```python
from build123d import *

# Parameters (mm, degrees)
SKETCH1_W           = 123.84
SKETCH1_H           = 33
BOSS_EXTRUDE1_DEPTH = 10
SKETCH2_W           = 12
SKETCH2_H           = 57
BOSS_EXTRUDE2_DEPTH = 70
SKETCH3_R           = 23.5
CUT_EXTRUDE1_DEPTH  = 124.84
SKETCH10_R          = 45
BOSS_EXTRUDE5_DEPTH = 10
SKETCH9_R           = 2.5
SKETCH9_W           = 10
SKETCH9_H           = 24
CUT_EXTRUDE3_DEPTH  = 21
FILLET1_R           = 28
SKETCH11_R          = 23.5
SKETCH11_R_2        = 20
BOSS_EXTRUDE6_DEPTH = 5
SKETCH12_R          = 23.5
SKETCH12_R_2        = 20
BOSS_EXTRUDE7_DEPTH = 5


with BuildPart() as part:
    # Sketch1 → Boss-Extrude1 (new body)
    with BuildSketch(Plane(origin=(0, 0, 0), x_dir=(1, 0, 0), z_dir=(0, 1, 0))):
        Rectangle(SKETCH1_W, SKETCH1_H)
    extrude(amount=BOSS_EXTRUDE1_DEPTH)

    # Sketch2 → Boss-Extrude2 (add)
    with BuildSketch(Plane(origin=(0, 10, 0), x_dir=(1, 0, 0), z_dir=(0, 1, 0))):
        with Locations((-55.92, 0)):
            Rectangle(SKETCH2_W, SKETCH2_H)
        with Locations((55.92, 0)):
            Rectangle(SKETCH2_W, SKETCH2_H)
    extrude(amount=BOSS_EXTRUDE2_DEPTH)

    # Sketch3 → Cut-Extrude1 (cut, through all)
    with BuildSketch(Plane(origin=(61.92, 0, 0), x_dir=(0, 0, -1), z_dir=(1, 0, 0))):
        with Locations((0, 49)):
            Circle(SKETCH3_R)
    extrude(amount=-CUT_EXTRUDE1_DEPTH, mode=Mode.SUBTRACT)

    # Sketch10 → Boss-Extrude5 (add)
    with BuildSketch(Plane.XZ):
        Circle(SKETCH10_R)
    extrude(amount=BOSS_EXTRUDE5_DEPTH)

    # Sketch9 → Cut-Extrude3 (cut, through all)
    with BuildSketch(Plane(origin=(0, 10, 0), x_dir=(1, 0, 0), z_dir=(0, 1, 0))):
        with Locations((21.118713953, -21.307273899)):
            Circle(SKETCH9_R)
        with Locations((21.307273899, 21.118713953)):
            Circle(SKETCH9_R)
        with Locations((-21.118713953, 21.307273899)):
            Circle(SKETCH9_R)
        with Locations((-28.5, 0)):
            Rectangle(SKETCH9_W, SKETCH9_H)
        with Locations((28.5, 0)):
            Rectangle(SKETCH9_W, SKETCH9_H)
    extrude(amount=-CUT_EXTRUDE3_DEPTH, mode=Mode.SUBTRACT)

    # Fillet1
    fillet1_edges = [part.edges().sort_by_distance(p)[0] for p in [
        (-55.92, 80, 28.5),
        (-55.92, 80, -28.5),
        (55.92, 80, -28.5),
        (55.92, 80, 28.5),
    ]]
    fillet(fillet1_edges, radius=FILLET1_R)

    # Sketch11 → Boss-Extrude6 (add)
    with BuildSketch(Plane(origin=(61.92, 0, 0), x_dir=(0, 0, -1), z_dir=(1, 0, 0))):
        with Locations((0, 49)):
            Circle(SKETCH11_R)
        with Locations((0, 49)):
            Circle(SKETCH11_R_2, mode=Mode.SUBTRACT)
    extrude(amount=-BOSS_EXTRUDE6_DEPTH)

    # Sketch12 → Boss-Extrude7 (add)
    with BuildSketch(Plane.ZY.offset(61.92)):
        with Locations((0, 49)):
            Circle(SKETCH12_R)
        with Locations((0, 49)):
            Circle(SKETCH12_R_2, mode=Mode.SUBTRACT)
    extrude(amount=-BOSS_EXTRUDE7_DEPTH)


solid = part.part
```
Geometry: final body of the model. Coordinates: model frame, mm. A direction names the side the tool comes from. Round coordinates to 2 decimals unless told otherwise and drop trailing zeros. Order: outer loops, then holes, each group sorted by start corner. A loop starts at its lowest first (then second) coordinate and runs counter-clockwise, first axis right, second up. Notation, with made-up numbers: (-37, 85) - (14, 85) arc R9 cw to (14, 95) - close; hole circle Ø6 at (74.25, -10). An arc over 180 degrees is marked (long way). Use CSV: the item, a comma, the result in double quotes. Start each with the question number.
Q1. Section query A-A (y = 13.5). Return loops of the section in (x, z), and give its area (3 significant figures).
Q2. Mould query, pull axis X, two halves, no side actions, for faces 1 (the face through (-61.92, 23, 0)), 2 (the face through (49.92, 29, 13)), 3 (the face through (56, 31, -28.5)). Classes: +X half, -X half, draft (parallel to the pull), parting line (faces both ways), or undercut.
Q3. Access query for faces 4 (the face through (-53.4, 56.1, -22.4)), 5 (the face through (56, 10, -23)), 6 (the face through (-1, 5, -16.5)), 7 (the face through (-33.5, 0, 0)). Directions: +Z, -Z, +X, -X, +Y, -Y. A direction counts if a zero-diameter tool reaches every point of the face in a straight line with its end or side. Return the directions, or none.
Q4. Material intervals for line 1 along X through (y, z) = (42.5, -23); line 2 along Y through (x, z) = (10, 41.5); line 3 along Z through (x, y) = (-51, 48), sorted ascending. Write a range as from..to.
Q5. Section query B-B (y = 49). Return loops of the section in (x, z), and give its area (3 significant figures).
Q6. Section query C-C (x = 22). Return loops of the section in (y, z).
Q7. Section query D-D (y = 4.5). Return loops of the section in (x, z), and give its area (3 significant figures).
Q8. First-contact query: pin 1 (13 mm diameter, centred on x = -57, z = 21.5, fed in from -Y); pin 2 (14.5 mm diameter, centred on x = -7.5, z = -30.5, fed in from +Y); pin 3 (16.5 mm diameter, centred on x = 15.5, z = -7, fed in from +Y). Flat tips, straight axial feed; report the tip coordinate or a pass-through.
Result set:
1,outline,"(-61.92, -28.5) - (-49.92, -28.5) - (-49.92, 28.5) - (-61.92, 28.5) - close; (49.92, -28.5) - (61.92, -28.5) - (61.92, 28.5) - (49.92, 28.5) - close"
1,area,"1,370 mm2"
2,face 1,"-X half"
2,face 2,"undercut"
2,face 3,"draft"
3,face 4,"none"
3,face 5,"-Z, +X, -X, -Y"
3,face 6,"-Z, +X, -X"
3,face 7,"+Y, -Y"
4,line 1,"x = -61.92..-49.92, 49.92..61.92"
4,line 2,"y = -10..0"
4,line 3,"z = -28.5..-23.48, 23.48..28.5"
5,outline,"(-61.92, -28.5) - (-49.92, -28.5) - (-49.92, -23.5) - (-56.92, -23.5) - (-56.92, -20) - (-61.92, -20) - close; (-61.92, 20) - (-56.92, 20) - (-56.92, 23.5) - (-49.92, 23.5) - (-49.92, 28.5) - (-61.92, 28.5) - close; (49.92, -28.5) - (61.92, -28.5) - (61.92, -20) - (56.92, -20) - (56.92, -23.5) - (49.92, -23.5) - close; (49.92, 23.5) - (56.92, 23.5) - (56.92, 20) - (61.92, 20) - (61.92, 28.5) - (49.92, 28.5) - close"
5,area,"310 mm2"
6,outline,"(-10, -39.26) - (0, -39.26) - (0, -23.52) - (-10, -23.52) - close; (-10, -18.72) - (0, -18.72) - (0, -16.5) - (10, -16.5) - (10, 16.5) - (0, 16.5) - (0, 18.97) - (-10, 18.97) - close; (-10, 23.65) - (0, 23.65) - (0, 39.26) - (-10, 39.26) - close"
7,outline,"(-61.92, -16.5) - (61.92, -16.5) - (61.92, 16.5) - (-61.92, 16.5) - close; hole (-33.5, -12) - (-23.5, -12) - (-23.5, 12) - (-33.5, 12) - close; hole (23.5, -12) - (33.5, -12) - (33.5, 12) - (23.5, 12) - close"
7,area,"3,610 mm2"
8,pin 1,"stops at y = 0"
8,pin 2,"stops at y = 0"
8,pin 3,"stops at y = 10"
